```python
from build123d import *

# Parameters (mm, degrees)
F0_W     = 100
F0_H     = 25
F2_DEPTH = 4
F3_W     = 40
F3_H     = 25
F4_DEPTH = 11
F5_W     = 9.8
F5_H     = 25
F6_DEPTH = 3
F9_D     = 3.2
F10_D    = 3.2
F12_D    = 8.5
F14_D    = 3.2


with BuildPart() as f2:
    # F0 (on Front) → F2 (new body)
    with BuildSketch(Plane.XZ):
        with Locations((-50, 12.5)):
            Rectangle(F0_W, F0_H)
    extrude(amount=F2_DEPTH)

    # F3 (on Front) → F4 (join)
    with BuildSketch(Plane.XZ):
        with Locations((-20, 12.5)):
            Rectangle(F3_W, F3_H)
    extrude(amount=F4_DEPTH)

    # F5 (on face) → F6 (join)
    with BuildSketch(Plane.XZ.offset(11)):
        with Locations((-19.9, 12.5)):
            Rectangle(F5_W, F5_H)
    extrude(amount=F6_DEPTH)

    # F9 (through all)
    with Locations(Plane.XZ.offset(4)):
        with Locations((-96, 22)):
            Hole(F9_D / 2)

    # F10 (through all)
    with Locations(Plane.XZ.offset(4)):
        with Locations((-76, 22)):
            Hole(F10_D / 2)

    # F12 (through all)
    with Locations(Plane.XZ.offset(14)):
        with Locations((-19.9, 12.5)):
            Hole(F12_D / 2)

    # F14 (through all)
    with Locations(Plane.XZ.offset(4)):
        with Locations((-96, 3), (-76, 3)):
            Hole(F14_D / 2)


solid = f2.part
```
Input: part model. Units: mm. Frame: model coordinates. A direction names the side the tool comes from. Coordinates: 2 decimals unless noted, no trailing zeros. Loops run counter-clockwise (first coordinate to the right, second up) from the corner with the lowest first, then second, coordinate; pieces in that order, holes last. Notation, with made-up numbers: M 12.5,-8.75 L 60.5,-8.75 A12 ccw 60.5,12.25 Z; hole C 59.25,-14.5 d8. An arc over 180 degrees is marked long. One line per item, written item: value.
(1) Section A-A (z = 12.5). Output: boundary loops of the cut face in (x, y).
Filled in:
outline: M -100,-4 L -40,-4 L -40,-11 L -24.8,-11 L -24.8,-14 L -24.15,-14 L -24.15,0 L -100,0 Z; M -15.65,-14 L -15,-14 L -15,-11 L 0,-11 L 0,0 L -15.65,0 Z
(2) Pull-direction query (Z, two-part tool) for faces 4 (the flat face through (-39.6, -5.3, 25)), 5 (the flat face through (-24.8, -12, 12)), 6 (the cylindrical face through (-94.4, -1.97, 3.07)); classes: +Z half, -Z half, draft (parallel to the pull), parting line (faces both ways), or undercut.
Filled in:
face 4: +Z half
face 5: draft
face 6: undercut
(3) Section C-C (y = -13). Output: boundary loops of the cut face in (x, z).
Filled in:
outline: M -24.8,0 L -15,0 L -15,25 L -24.8,25 Z; hole C -19.9,12.5 d8.5
(4) Line query: line 1 along Z through (x, y) = (-76, -2.05); line 2 along X through (y, z) = (-2, 4); line 3 along Y through (x, z) = (-37, 18). Output: solid intervals per line, ascending. Write a range as from..to.
Filled in:
line 1: 0..1.4, 4.6..20.4, 23.6..25
line 2: -100..-97.25, -94.75..-77.25, -74.75..0
line 3: -11..0
(5) Pin query (flat end, axial travel): pin 1 (5 mm diameter, centred on x = -76, z = 3, fed in from +Y); pin 2 (0.9 mm diameter, centred on y = -13, z = 14, fed in from -X); pin 3 (7.5 mm diameter, centred on x = -10.5, z = 14.5, fed in from -Y); pin 4 (6 mm diameter, centred on x = -58.5, z = 5.5, fed in from -Y). Return the tip coordinate at first contact, or that it passes through.
Filled in:
pin 1: y = 0
pin 2: x = -24.8
pin 3: y = -11
pin 4: y = -4
(6) Reachability of faces 1 (the flat face through (-40, -7, 12)), 2 (the flat face through (-15, -12, 12)), 3 (the cylindrical face through (-77.526, -1.972, 22.481)) from +Z, -Z, +X, -X, +Y, -Y: full face, straight path, thin tool, end or side. Return the list, or none.
Filled in:
face 1: +Z, -Z, -X, -Y
face 2: +Z, -Z, +X, -Y
face 3: +Y, -Y
(7) Section B-B (x = -96). Output: boundary loops of the cut face in (y, z), and give its area (3 significant figures).
Filled in:
outline: M -4,0 L 0,0 L 0,1.4 L -4,1.4 Z; M -4,4.6 L 0,4.6 L 0,20.4 L -4,20.4 Z; M -4,23.6 L 0,23.6 L 0,25 L -4,25 Z
area: 74.4 mm^2
(8) Section D-D (z = 22). Output: boundary loops of the cut face in (x, y), and give its area (3 significant figures).
Filled in:
outline: M -100,-4 L -97.6,-4 L -97.6,0 L -100,0 Z; M -94.4,-4 L -77.6,-4 L -77.6,0 L -94.4,0 Z; M -74.4,-4 L -40,-4 L -40,-11 L -24.8,-11 L -24.8,-14 L -15,-14 L -15,-11 L 0,-11 L 0,0 L -74.4,0 Z
area: 684 mm^2
